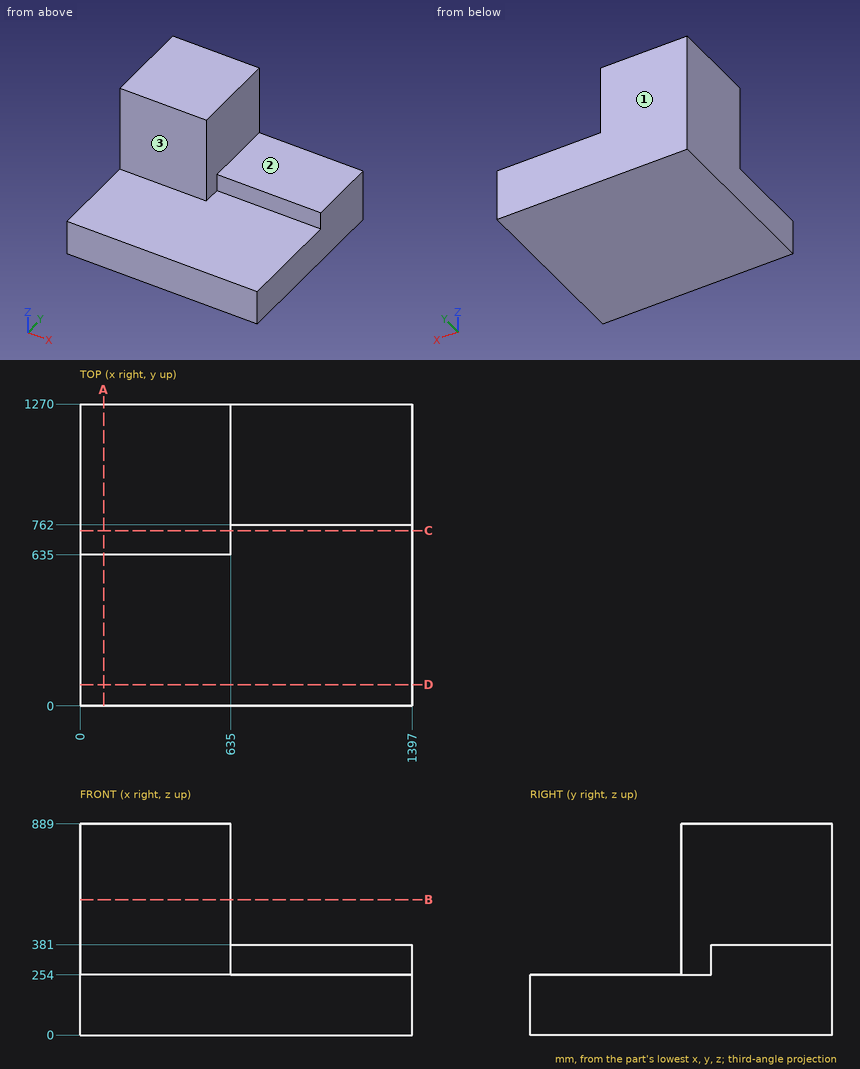
Answer from the drawing. Dimensions are ordinates in mm from the lowest x, y and z of the part. A direction names the side the tool comes from. Coordinates: 2 decimals unless noted, no trailing zeros. Order: outer loops, then holes, each group sorted by start corner. A loop starts at its lowest first (then second) coordinate and runs counter-clockwise, first axis right, second up. Notation, with made-up numbers: (6, 8) - (36, 8) arc R18 cw to (36, 26) - close; hole circle Ø5 at (-39, 78). An arc over 180 degrees is marked (long way). Put each result on its own line as item: value. Start each with the question number.
1) Find section D-D (y = 89). Give the vertices of the cut face in (x, z).
2) Find section C-C (y = 737.5). Give the vertices of the cut face in (x, z), plus the area to 3 significant figures.
3) Find section B-B (z = 570.5). Give the vertices of the cut face in (x, y).
4) Flat-ended cylindrical pins translate along their axes: pin 1 (3 mm diameter, centred on x = 377.5, y = 147.5, fed in from -Z); pin 2 (5 mm diameter, centred on x = 496.5, z = 301, fed in from -Y); pin 3 (6 mm diameter, centred on x = 844.5, y = 785.5, fed in from +Z); pin 4 (1.5 mm diameter, centred on y = 705, z = 589, fed in from +X). Find the tip coordinate at first contact, or state that the pin passes through.
5) Find the intervals of material crossed by line 1 (Z direction, x = 375, y = 564); line 2 (Y direction, x = 82, z = 655); line 3 (Y direction, x = 1140, z = 343.5), in increasing order. Write a range as from..to.
6) For the marked faces 1, 2 and 3, determine the directions among +Z, -Z, +X, -X, +Y, -Y from which every point of the face is accessible in a straight line to the end or side of a thin tool.
7) Find section A-A (x = 99). Give the vertices of the cut face in (y, z), plus the area to 3 significant figures.
Results list:
1. outline: (0, 0) - (1397, 0) - (1397, 254) - (0, 254) - close
2. outline: (0, 0) - (1397, 0) - (1397, 254) - (635, 254) - (635, 889) - (0, 889) - close
2. area: 758,000 mm^2
3. outline: (0, 635) - (635, 635) - (635, 1270) - (0, 1270) - close
4. pin 1: stops at z = 0
4. pin 2: stops at y = 635
4. pin 3: stops at z = 381
4. pin 4: stops at x = 635
5. line 1: z = 0..254
5. line 2: y = 635..1270
5. line 3: y = 762..1270
6. face 1: +Z, -Z, +X, -X, +Y
6. face 2: +Z, +X, +Y, -Y
6. face 3: +Z, +X, -X, -Y
7. outline: (0, 0) - (1270, 0) - (1270, 889) - (635, 889) - (635, 254) - (0, 254) - close
7. area: 726,000 mm^2
